For this review, take the finished solid that the model builds, in its own axes (mm). A direction names the side the tool comes from. Coordinates: 2 decimals unless noted, no trailing zeros. Loops run counter-clockwise (first coordinate to the right, second up) from the corner with the lowest first, then second, coordinate; pieces in that order, holes last. Notation, with made-up numbers: M -36.75,-0.75 L 2.25,-0.75 A25 ccw 2.25,11.25 Z; hole C -17.75,-18.75 d9. An arc over 180 degrees is marked long. Answer as a JSON object with one key per item and string values. Group by question number.
Item 1: Add section C-C (z = 17). State the section outline as (x, y) points.
Item 2: Add section D-D (x = 1.65). State the section outline as (y, z) points.
Item 3: Add section B-B (y = -1.2). State the section outline as (x, z) points, then the cut area to 3 significant figures.
Item 4: Tool access review of faces 1 (the face through (0, -2, 16)), 2 (the face through (0, 1, 28)), 3 (the face through (0, 0, 2)): name each direction out of +Z, -Z, +X, -X, +Y, -Y from which nothing blocks a thin tool from reaching the whole face with its end or side.
Item 5: Insertion check: pin 1 (1 mm diameter, centred on x = -1, y = 1, fed in from -Z); pin 2 (2 mm diameter, centred on x = 1, z = 30.5, fed in from +Y). Each pin has a flat end and moves straight along its axis. Give the tip position at first contact, or say it passes through.
Item 6: Wall thickness on L1, parallel to Z at x = -1, y = 0.6; L2, parallel to Y at x = 0.1, z = 24.5; L3, parallel to Y at x = -0.05, z = 3.5: over which ranges is each line inside the solid? List them lowest first. Write a range as from..to.
Item 7: Add section A-A (x = 0). State the section outline as (y, z) points, then the cut area to 3 significant figures.
from build123d import *

# Parameters (mm, degrees)
ESQUISSE1_R             = 2
BOSS_EXTRU_1_DEPTH      = 33
ESQUISSE2_W             = 4
ESQUISSE2_H             = 3
ENL_V_MAT_EXTRU_1_DEPTH = 5


with BuildPart() as part:
    # Esquisse1 → Boss.-Extru.1 (new body)
    with BuildSketch(Plane.XY):
        Circle(ESQUISSE1_R)
    extrude(amount=BOSS_EXTRU_1_DEPTH)

    # Esquisse2 → Enlèv. mat.-Extru.1 (cut)
    with BuildSketch(Plane(origin=(0, 0, 0), x_dir=(-1, 0, 0), z_dir=(0, 0, -1))):
        with Locations((0, 1.5)):
            Rectangle(ESQUISSE2_W, ESQUISSE2_H)
    enl_v_mat_extru_1 = extrude(amount=-ENL_V_MAT_EXTRU_1_DEPTH, mode=Mode.SUBTRACT)

    # Symétrie1: Enlèv. mat.-Extru.1 across plane
    add(enl_v_mat_extru_1.mirror(Plane.XY.offset(16.5)), mode=Mode.SUBTRACT)


solid = part.part
From the geometry:
{
 "1": {"outline": "C 0,0 d4"},
 "2": {"outline": "M -1.13,0 L 0,0 L 0,5 L 1.13,5 L 1.13,28 L 0,28 L 0,33 L -1.13,33 Z"},
 "3": {"outline": "M -1.6,0 L 1.6,0 L 1.6,33 L -1.6,33 Z", "area": "106 mm²"},
 "4": {"face 1": "+Z, -Z", "face 2": "+Z, +X, -X, +Y", "face 3": "-Z, +X, -X, +Y"},
 "5": {"pin 1": "stops at z = 5", "pin 2": "stops at y = 0"},
 "6": {"L1": "z = 5..28", "L2": "y = -2..2", "L3": "y = -2..0"},
 "7": {"outline": "M -2,0 L 0,0 L 0,5 L 2,5 L 2,28 L 0,28 L 0,33 L -2,33 Z", "area": "112 mm²"}
}
